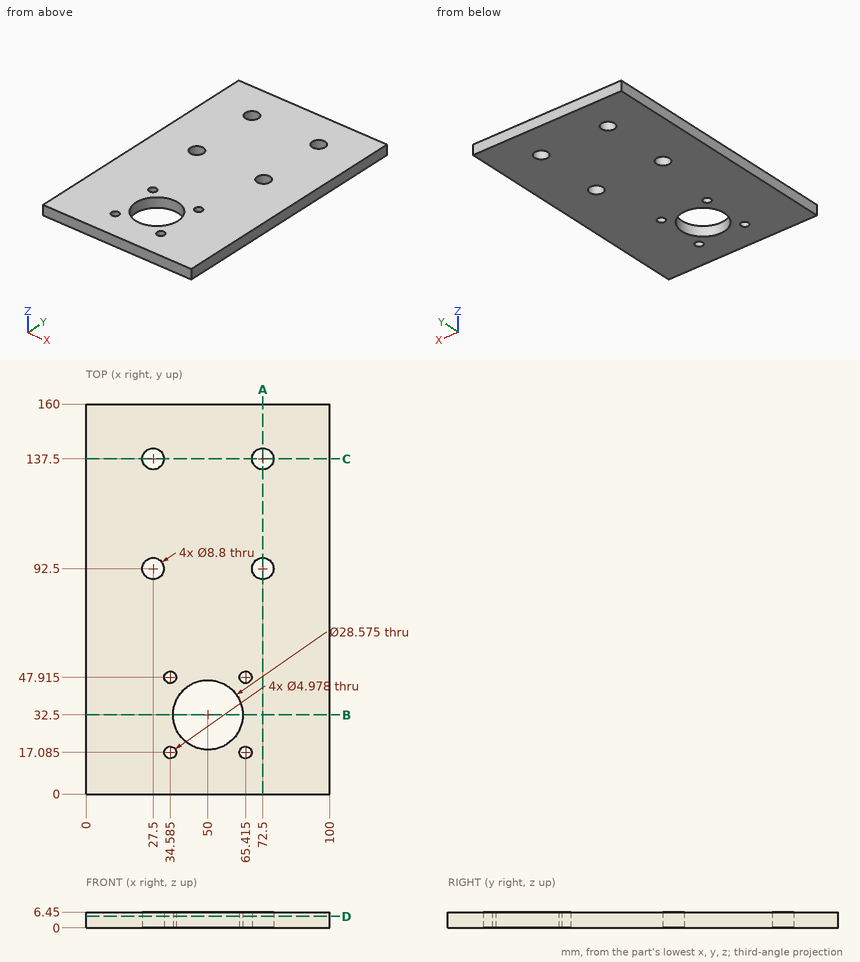
The figure shows three views and two pictorial views of one solid part (mm, origin at its lowest corner). Answer the questions. Give positions to 0.01 mm unless a question says otherwise; leave off trailing zeros. Order: outer loops, then holes, each group sorted by start corner. A loop starts at its lowest first (then second) coordinate and runs counter-clockwise, first axis right, second up. Notation, with made-up numbers: (64.5, 32) -> (79.5, 32) arc R15 cw to (79.5, 36) -> close; hole circle Ø3 at (74, 25). An arc over 180 degrees is marked (long way). Answer as CSV lines item,"result". Start each with the question number.
(1) This flat-tipped pin is pushed along its axis until it touches: pin 1 Ø12 at (x, y) = (59, 58) entering from -Z. Where does it stop, or does it pass through?
(2) Section A-A, the plane x = 72.5 is taken. Write down the section's boundary in (y, z).
(3) Section C-C, the plane y = 137.5 is taken. Write down the section's boundary in (x, z).
(4) Section D-D, the plane z = 4.75 is taken. Give the number of separate pieces and of enclosed holes in the cut face, plus the area to 3 significant figures.
(5) Section B-B, the plane y = 32.5 is taken. Write down the section's boundary in (x, z), plus the area to 3 significant figures.
(6) Consider line 1 along Y through (x, z) = (50, 3); line 2 along Y through (x, z) = (31, 3.5) (1 decimal); line 3 along X through (y, z) = (18, 5.25). Determine where each line is inside the solid, lowest interval first.
Entries:
1,pin 1,"z = 0"
2,outline,"(0, 0) -> (88.1, 0) -> (88.1, 6.45) -> (0, 6.45) -> close; (96.9, 0) -> (133.1, 0) -> (133.1, 6.45) -> (96.9, 6.45) -> close; (141.9, 0) -> (160, 0) -> (160, 6.45) -> (141.9, 6.45) -> close"
3,outline,"(0, 0) -> (23.1, 0) -> (23.1, 6.45) -> (0, 6.45) -> close; (31.9, 0) -> (68.1, 0) -> (68.1, 6.45) -> (31.9, 6.45) -> close; (76.9, 0) -> (100, 0) -> (100, 6.45) -> (76.9, 6.45) -> close"
4,separate pieces,"1"
4,enclosed holes,"9"
4,area,"15,000 mm²"
5,outline,"(0, 0) -> (35.71, 0) -> (35.71, 6.45) -> (0, 6.45) -> close; (64.29, 0) -> (100, 0) -> (100, 6.45) -> (64.29, 6.45) -> close"
5,area,"461 mm²"
6,line 1,"0 to 18.21, 46.79 to 160"
6,line 2,"0 to 89.8, 95.2 to 134.8, 140.2 to 160"
6,line 3,"0 to 32.27, 36.9 to 63.1, 67.73 to 100"
